```python
from build123d import *

# Parameters (mm, degrees)
CROQUIS1_W                 = 265.5
CROQUIS1_H                 = 142
CROQUIS1_W_2               = 235.5
CROQUIS1_H_2               = 112
SALIENTE_EXTRUIR1_DEPTH    = 3
SALIENTE_EXTRUIR2_DEPTH    = 20
SIMETR_A2_COPY_1_DEPTH     = 20
SALIENTE_EXTRUIR3_DEPTH    = 10
CROQUIS5_W                 = 38.206392887
CROQUIS5_H                 = 90
CORTAR_EXTRUIR2_DEPTH      = 160.539376017
CROQUIS6_W                 = 15
CROQUIS6_H                 = 112
SALIENTE_EXTRUIR4_DEPTH    = 3
CROQUIS8_W                 = 31
CROQUIS8_H                 = 4.5
CORTAR_EXTRUIR4_DEPTH      = 3
CROQUIS9_R                 = 1.75
CORTAR_EXTRUIR5_DEPTH      = 160.539376017
CROQUIS11_R                = 1.75
CORTAR_EXTRUIR7_DEPTH      = 4
CROQUIS12_R                = 1.75
CORTAR_EXTRUIR8_DEPTH      = 4
REDONDEO1_R                = 7
REDONDEO2_R                = 7
CROQUIS13_R                = 1.75
CORTAR_EXTRUIR9_DEPTH      = 159.964815289
CROQUIS15_R                = 1.75
CORTAR_EXTRUIR10_DEPTH     = 159.964815289
SIMETR_A12_COPY_1_SKETCH_R = 1.75
SIMETR_A12_COPY_1_DEPTH    = 159.964815289
REDONDEO3_R                = 7


with BuildPart() as part:
    # Croquis1 → Saliente-Extruir1 (new body)
    with BuildSketch(Plane(origin=(0, 0, 0), x_dir=(1, 0, 0), z_dir=(0, 1, 0))):
        Rectangle(CROQUIS1_W, CROQUIS1_H)
        Rectangle(CROQUIS1_W_2, CROQUIS1_H_2, mode=Mode.SUBTRACT)
    extrude(amount=SALIENTE_EXTRUIR1_DEPTH)

    # Croquis2 → Saliente-Extruir2 (add)
    with BuildSketch(Plane.ZY.offset(127.25)):
        Polygon((66.5, 0), (66.5, -26), (82.5, -26), (82.5, -29), (63.5, -29), (63.5, 0), align=None)
    saliente_extruir2 = extrude(amount=-SALIENTE_EXTRUIR2_DEPTH)

    # Simetría1: Saliente-Extruir2 across plane
    add(saliente_extruir2.mirror(Plane(origin=(0, 0, 0), x_dir=(0, 0, 1), z_dir=(1, 0, 0))))

    # Simetría2: Saliente-Extruir2 across plane
    add(saliente_extruir2.mirror(Plane.XY))

    # Simetría2 copy 1 sketch → Simetría2 copy 1 (add)
    with BuildSketch(Plane(origin=(127.25, 0, 0), x_dir=(0, 0, -1), z_dir=(1, 0, 0))):
        Polygon((66.5, 0), (66.5, -26), (82.5, -26), (82.5, -29), (63.5, -29), (63.5, 0), align=None)
    extrude(amount=-SIMETR_A2_COPY_1_DEPTH)

    # Croquis4 → Saliente-Extruir3 (add, symmetric)
    with BuildSketch(Plane(origin=(-36.45, 0, 0), x_dir=(0, 0, -1), z_dir=(1, 0, 0))):
        Polygon((-82.5, -29), (-63.5, -29), (-63.5, 0), (-66.5, 0), (-66.5, -26), (-82.5, -26), align=None)
    saliente_extruir3 = extrude(amount=SALIENTE_EXTRUIR3_DEPTH, both=True)

    # Simetría4: Saliente-Extruir3 across plane
    add(saliente_extruir3.mirror(Plane.XY))

    # Croquis5 → Cortar-Extruir2 (cut, through all)
    with BuildSketch(Plane(origin=(0, 3, 0), x_dir=(1, 0, 0), z_dir=(0, 1, 0))):
        with Locations((-124.602228384, 0)):
            Rectangle(CROQUIS5_W, CROQUIS5_H)
    extrude(amount=-CORTAR_EXTRUIR2_DEPTH, mode=Mode.SUBTRACT)

    # Croquis6 → Saliente-Extruir4 (add)
    with BuildSketch(Plane(origin=(0, 3, 0), x_dir=(1, 0, 0), z_dir=(0, 1, 0))):
        with Locations((-36.45, 0)):
            Rectangle(CROQUIS6_W, CROQUIS6_H)
    extrude(amount=-SALIENTE_EXTRUIR4_DEPTH)

    # Croquis8 → Cortar-Extruir4 (cut)
    with BuildSketch(Plane(origin=(0, 3, 0), x_dir=(1, 0, 0), z_dir=(0, 1, 0))):
        with Locations((97.85, 68.75)):
            Rectangle(CROQUIS8_W, CROQUIS8_H)
        with Locations((-57.45, 68.75)):
            Rectangle(CROQUIS8_W, CROQUIS8_H)
    cortar_extruir4 = extrude(amount=-CORTAR_EXTRUIR4_DEPTH, mode=Mode.SUBTRACT)

    # Croquis9 → Cortar-Extruir5 (cut, through all)
    with BuildSketch(Plane(origin=(0, 3, 0), x_dir=(1, 0, 0), z_dir=(0, 1, 0))):
        with Locations(Location((-127.25, 59, 0), (0, 0, 270))):
            Circle(CROQUIS9_R)
        with Locations(Location((-127.25, 50.2, 0), (0, 0, 270))):
            Circle(CROQUIS9_R)
    cortar_extruir5 = extrude(amount=-CORTAR_EXTRUIR5_DEPTH, mode=Mode.SUBTRACT)

    # Croquis11 → Cortar-Extruir7 (cut)
    with BuildSketch(Plane(origin=(0, 3, 0), x_dir=(1, 0, 0), z_dir=(0, 1, 0))):
        with Locations(Location((103.750895814, 61.952994616, 0), (0, 0, 270))):
            Circle(CROQUIS11_R)
        with Locations(Location((94.950895814, 61.952994616, 0), (0, 0, 270))):
            Circle(CROQUIS11_R)
    cortar_extruir7 = extrude(amount=-CORTAR_EXTRUIR7_DEPTH, mode=Mode.SUBTRACT)

    # Croquis12 → Cortar-Extruir8 (cut)
    with BuildSketch(Plane(origin=(0, 3, 0), x_dir=(1, 0, 0), z_dir=(0, 1, 0))):
        with Locations(Location((-51.449104186, 61.952994616, 0), (0, 0, 270))):
            Circle(CROQUIS12_R)
        with Locations(Location((-60.249104186, 61.952994616, 0), (0, 0, 270))):
            Circle(CROQUIS12_R)
    cortar_extruir8 = extrude(amount=-CORTAR_EXTRUIR8_DEPTH, mode=Mode.SUBTRACT)

    # Simetría5: Cortar-Extruir5, Cortar-Extruir7, Cortar-Extruir8 across plane
    add(cortar_extruir5.mirror(Plane.XY), mode=Mode.SUBTRACT)
    add(cortar_extruir7.mirror(Plane.XY), mode=Mode.SUBTRACT)
    add(cortar_extruir8.mirror(Plane.XY), mode=Mode.SUBTRACT)

    # Simetría6: Cortar-Extruir4 across plane
    add(cortar_extruir4.mirror(Plane.XY), mode=Mode.SUBTRACT)

    # Redondeo1
    redondeo1_edges = [part.edges().sort_by_distance(p)[0] for p in [
        (-107.25, -27.5, 82.5),
        (-127.25, -27.5, 82.5),
    ]]
    fillet(redondeo1_edges, radius=REDONDEO1_R)

    # Redondeo2
    redondeo2_edges = [part.edges().sort_by_distance(p)[0] for p in [
        (-46.45, -27.5, 82.5),
        (-26.45, -27.5, 82.5),
        (127.25, -27.5, 82.5),
        (107.25, -27.5, 82.5),
    ]]
    fillet(redondeo2_edges, radius=REDONDEO2_R)

    # Croquis13 → Cortar-Extruir9 (cut, through all)
    with BuildSketch(Plane(origin=(0, -26, 0), x_dir=(1, 0, 0), z_dir=(0, 1, 0))):
        with Locations(Location((-117.25, -73.5, 0), (0, 0, 270))):
            Circle(CROQUIS13_R)
    cortar_extruir9 = extrude(amount=-CORTAR_EXTRUIR9_DEPTH, mode=Mode.SUBTRACT)

    # Simetría7: Cortar-Extruir9 across plane
    add(cortar_extruir9.mirror(Plane(origin=(0, 0, 0), x_dir=(0, 0, 1), z_dir=(1, 0, 0))), mode=Mode.SUBTRACT)

    # Croquis15 → Cortar-Extruir10 (cut, through all)
    with BuildSketch(Plane(origin=(0, -26, 0), x_dir=(1, 0, 0), z_dir=(0, 1, 0))):
        with Locations(Location((-36.45, -73.5, 0), (0, 0, 270))):
            Circle(CROQUIS15_R)
    cortar_extruir10 = extrude(amount=-CORTAR_EXTRUIR10_DEPTH, mode=Mode.SUBTRACT)

    # Simetría12: Cortar-Extruir9, Cortar-Extruir10 across plane
    add(cortar_extruir9.mirror(Plane.XY), mode=Mode.SUBTRACT)
    add(cortar_extruir10.mirror(Plane.XY), mode=Mode.SUBTRACT)

    # Simetría12 copy 1 sketch → Simetría12 copy 1 (cut, through all)
    with BuildSketch(Plane(origin=(0, -26, 0), x_dir=(-1, 0, 0), z_dir=(0, 1, 0))):
        with Locations(Location((-117.25, -73.5, 0), (0, 0, 270))):
            Circle(SIMETR_A12_COPY_1_SKETCH_R)
    extrude(amount=-SIMETR_A12_COPY_1_DEPTH, mode=Mode.SUBTRACT)

    # Redondeo3
    redondeo3_edges = [part.edges().sort_by_distance(p)[0] for p in [
        (-26.45, -27.5, -82.5),
        (-46.45, -27.5, -82.5),
        (107.25, -27.5, -82.5),
        (127.25, -27.5, -82.5),
        (-127.25, -27.5, -82.5),
        (-107.25, -27.5, -82.5),
    ]]
    fillet(redondeo3_edges, radius=REDONDEO3_R)


solid = part.part
```
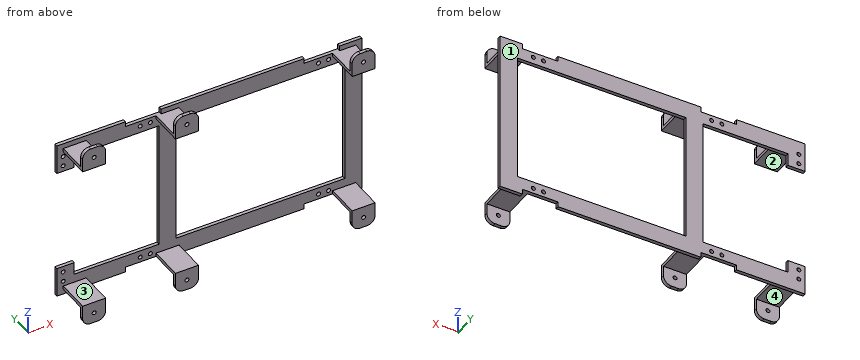
Input: part model. Units: mm. Frame: model coordinates. Face numbers are marked on the shaded views. Coordinates: 2 decimals unless noted, no trailing zeros. Loops run counter-clockwise (first coordinate to the right, second up) from the corner with the lowest first, then second, coordinate; pieces in that order, holes last. Notation, with made-up numbers: M 10.5,37.5 L 61.5,37.5 A25 ccw 61.5,69.5 Z; hole C -23,43 d4. An arc over 180 degrees is marked long. Answer in a Markdown table with one row per item.
1. Draft query along Z for the marked faces 1, 2, 3 and 4. Return one class per face: pulls with the +Z half, pulls with the -Z half, needs draft (parallel to the pull), parting line crosses it, or undercut.
Response:
| item | result |
|---|---|
| face 1 | needs draft |
| face 2 | undercut |
| face 3 | undercut |
| face 4 | pulls with the -Z half |
2. Section C-C, the plane y = -7. Output: boundary loops of the cut face in (x, z).
Response:
| item | result |
|---|---|
| outline | M -127.25,-66.5 L -107.25,-66.5 L -107.25,-63.5 L -127.25,-63.5 Z; M -127.25,63.5 L -107.25,63.5 L -107.25,66.5 L -127.25,66.5 Z; M -46.45,-66.5 L -26.45,-66.5 L -26.45,-63.5 L -46.45,-63.5 Z; M -46.45,63.5 L -26.45,63.5 L -26.45,66.5 L -46.45,66.5 Z; M 107.25,-66.5 L 127.25,-66.5 L 127.25,-63.5 L 107.25,-63.5 Z; M 107.25,63.5 L 127.25,63.5 L 127.25,66.5 L 107.25,66.5 Z |
3. First-contact query: pin 1 (10 mm diameter, centred on x = -121, y = -8, fed in from -Z); pin 2 (3.5 mm diameter, centred on x = -71.5, y = 2, fed in from +Z); pin 3 (12 mm diameter, centred on y = -1, z = 25, fed in from -X); pin 4 (2 mm diameter, centred on x = 94.95, z = -61.95, fed in from +Y). Flat tips, straight axial feed; report the tip coordinate or a pass-through.
Response:
| item | result |
|---|---|
| pin 1 | stops at z = -66.5 |
| pin 2 | stops at z = 71 |
| pin 3 | stops at x = -43.95 |
| pin 4 | passes through |
4. Section B-B, the plane x = -19.5. Output: boundary loops of the cut face in (y, z), then the cut area to 3 significant figures.
Response:
| item | result |
|---|---|
| outline | M 0,-71 L 3,-71 L 3,-56 L 0,-56 Z; M 0,56 L 3,56 L 3,71 L 0,71 Z |
| area | 90.0 mm2 |
5. Material intervals for line 1 (X direction, y = 2.4, z = -50.2); line 2 (Z direction, x = -32.5, y = -2); line 3 (Y direction, x = -35.5, z = 28), sorted ascending.
Response:
| item | result |
|---|---|
| line 1 | x = -132.75 to -129, -125.5 to -117.75, -43.95 to -28.95, 117.75 to 132.75 |
| line 2 | z = -66.5 to -63.5, 63.5 to 66.5 |
| line 3 | y = 0 to 3 |
6. Section A-A, the plane z = -17.5. Output: boundary loops of the cut face in (x, y), then the cut area to 3 significant figures.
Response:
| item | result |
|---|---|
| outline | M -43.95,0 L -28.95,0 L -28.95,3 L -43.95,3 Z; M 117.75,0 L 132.75,0 L 132.75,3 L 117.75,3 Z |
| area | 90.0 mm2 |
